```python
from build123d import *

# Parameters (mm, degrees)
F0_W      = 12.065
F0_H      = 12.065
F1_DEPTH  = 56.642
F2_W      = 15.0622
F2_H      = 15.0622
F2_W_2    = 12.065
F2_H_2    = 12.065
F3_DEPTH  = 37.3126
F4_W      = 15.0622
F4_H      = 3.1496
F5_DEPTH  = 37.3126
F6_W      = 9.2009786564
F6_H      = 3.1496
F7_DEPTH  = 254
F8_R      = 0.254
F9_R      = 1.27
F10_W     = 8.0772
F10_H     = 9.779
F11_DEPTH = 10.0584
F12_R     = 2.125
F13_DEPTH = 25
F14_R     = 3.5
F16_R     = 2.125
F17_DEPTH = 3


with BuildPart() as f1:
    # F0 (on Front) → F1 (new body)
    with BuildSketch(Plane.XZ):
        Rectangle(F0_W, F0_H)
    extrude(amount=F1_DEPTH)

    # F2 (on face) → F3 (join)
    with BuildSketch(Plane.XZ.offset(56.642)):
        Rectangle(F2_W, F2_H)
        Rectangle(F2_W_2, F2_H_2, mode=Mode.SUBTRACT)
        Rectangle(F2_W_2, F2_H_2)
    extrude(amount=F3_DEPTH)

    # F4 (on face) → F5 (join, through all)
    with BuildSketch(Plane(origin=(0, -56.642, 0), x_dir=(-1, 0, 0), z_dir=(0, 1, 0))):
        with Locations((0, 9.1059)):
            Rectangle(F4_W, F4_H)
    extrude(amount=-F5_DEPTH)

    # F6 (on face) → F7 (cut)
    with BuildSketch(Plane.YZ.offset(7.5311)):
        with Locations((-61.2424893282, 9.1059)):
            Rectangle(F6_W, F6_H)
    extrude(amount=-F7_DEPTH, mode=Mode.SUBTRACT)

    # F8
    f8_edges = [f1.edges().sort_by_distance(p)[0] for p in [
        (0, -56.642, 7.5311),
        (7.5311, -56.642, 0),
        (0, -56.642, -7.5311),
        (-7.5311, -56.642, 0),
        (-6.0325, 0, 0),
        (0, 0, 6.0325),
        (6.0325, 0, 0),
        (0, 0, -6.0325),
    ]]
    fillet(f8_edges, radius=F8_R)

    # F9
    f9_edges = [f1.edges().sort_by_distance(p)[0] for p in [
        (0, -65.842979, 10.6807),
        (0, -93.9546, 10.6807),
        (0, -93.9546, -7.5311),
    ]]
    fillet(f9_edges, radius=F9_R)

    # F10 (on face) → F11 (join)
    with BuildSketch(Plane.XZ.offset(93.9546)):
        Rectangle(F10_W, F10_H)
    extrude(amount=F11_DEPTH)

    # F12 (on face) → F13 (cut)
    with BuildSketch(Plane(origin=(-4.0386, 0, 0), x_dir=(0, -1, 0), z_dir=(-1, 0, 0))):
        with Locations((98.4546, 0)):
            Circle(F12_R)
    extrude(amount=-F13_DEPTH, mode=Mode.SUBTRACT)

    # F14
    f14_edges = [f1.edges().sort_by_distance(p)[0] for p in [
        (0, -104.013, 4.8895),
        (0, -104.013, -4.8895),
    ]]
    fillet(f14_edges, radius=F14_R)

    # F16 (on Right) → F17 (join, symmetric)
    with BuildSketch(Plane.YZ):
        with BuildLine():
            Line((0, 4.4995), (0, -4.5005))
            Line((0, -4.5005), (6, -4.5005))
            ThreePointArc((6, -4.5005), (6.7071067812, -4.2076067812), (7, -3.5005))
            Line((7, -3.5005), (7, 3.4995))
            ThreePointArc((7, 3.4995), (6.7071067812, 4.2066067812), (6, 4.4995))
            Line((6, 4.4995), (0, 4.4995))
        make_face()
        with Locations((4, 0)):
            Circle(F16_R, mode=Mode.SUBTRACT)
    extrude(amount=F17_DEPTH, both=True)


solid = f1.part
```
Geometry: final body of the model. Coordinates: model frame, mm. A direction names the side the tool comes from. Round coordinates to 2 decimals unless told otherwise and drop trailing zeros. Loops run counter-clockwise (first coordinate to the right, second up) from the corner with the lowest first, then second, coordinate; pieces in that order, holes last.
Item 1: Section B-B, the plane z = 0. State how many separate pieces and enclosed holes the cut face has, plus the area to 3 significant figures.
Checked values:
separate pieces: 3
enclosed holes: 0
area: 1,310 mm2
Item 2: Reachability of faces 1 (the flat face through (0, -61, 7.531)), 2 (the flat face through (0, -97, 4.89)), 3 (the flat face through (0, -28, -6.032)), 4 (the flat face through (4.039, -98.91, -2.24)), 5 (the flat face through (0, -97, -4.89)) from +Z, -Z, +X, -X, +Y, -Y: full face, straight path, thin tool, end or side. Return the list, or none.
Checked values:
face 1: +Z, +X, -X, +Y
face 2: +Z, +X, -X, -Y
face 3: -Z, +X, -X, +Y
face 4: +Z, -Z, +X, -Y
face 5: -Z, +X, -X, -Y
Item 3: Section D-D, the plane y = -61.5. Output: boundary loops of the cut face in (x, z), plus the area to 3 significant figures.
Checked values:
outline: (-7.53, -7.53) - (7.53, -7.53) - (7.53, 7.53) - (-7.53, 7.53) - close
area: 227 mm2
Item 4: Section C-C, the plane y = -35.5. Output: boundary loops of the cut face in (x, z), plus the area to 3 significant figures.
Checked values:
outline: (-6.03, -6.03) - (6.03, -6.03) - (6.03, 6.03) - (-6.03, 6.03) - close
area: 146 mm2
Item 5: Mould query, pull axis Y, two halves, no side actions, for faces 6 (the flat face through (0, 3, -4.5)), 7 (the cylindrical face through (0.06, -102.96, 3.89)), 8 (the cylindrical face through (0, 2.4, 1.4)). Classes: released by +Y, released by -Y, zero draft, split by the parting line, or undercut.
Checked values:
face 6: zero draft
face 7: released by -Y
face 8: undercut
Item 6: Line query: L1, parallel to Z at x = -0.55, y = 4 (1 decimal); L2, parallel to Z at x = -2, y = -23.5. Output: solid intervals per line, ascending.
Checked values:
L1: z = -4.5 to -2.1, 2.1 to 4.5
L2: z = -6.03 to 6.03
Item 7: Section A-A, the plane y = 4. Output: boundary loops of the cut face in (x, z) (1 decimal).
Checked values:
outline: (-3, -4.5) - (3, -4.5) - (3, -2.1) - (-3, -2.1) - close; (-3, 2.1) - (3, 2.1) - (3, 4.5) - (-3, 4.5) - close
Item 8: Contact query for flat-ended pins moving along their axis: P1, Ø5, axis at x = -1.5, y = -97, coming from the -Z side; P2, Ø5, axis at x = 1, y = -98, coming from the +Z side; P3, Ø5.5, axis at y = 4.5, z = -1.5, coming from the +X side. Output: stop coordinate, or through.
Checked values:
P1: stops at z = -4.89
P2: stops at z = 4.89
P3: stops at x = 3
